Geometry: final body of the model. Coordinates: model frame, mm. Face numbers are marked on the shaded views. Coordinates: 2 decimals unless noted, no trailing zeros. Order: outer loops, then holes, each group sorted by start corner. A loop starts at its lowest first (then second) coordinate and runs counter-clockwise, first axis right, second up. Notation, with made-up numbers: M 62,-12.75 L 90,-12.75 A29 cw 90,9.25 Z; hole C -24,38 d6. An arc over 180 degrees is marked long. Use CSV: the item, a comma, the result in double quotes. Start each with the question number.
1. Section query A-A on x = 266. Return the cut outline in (y, z), and give its area (3 significant figures).
2. First-contact query: P1, Ø10, axis at y = -292.5, z = -432, coming from the +X side; P2, Ø1.5, axis at x = 195, y = -426.5, coming from the -Z side; P3, Ø3, axis at y = 471, z = -355, coming from the -X side. Flat tips, straight axial feed; report the tip coordinate or a pass-through.
3. Material intervals for line 1 (X direction, y = -71, z = -378.5); line 2 (Y direction, x = 176.5, z = -317); line 3 (X direction, y = -426.5, z = -334), sorted ascending.
4. Pull-direction query (Y, two-part tool) for the marked faces 1, 2 and 3; classes: pulls with the +Y half, pulls with the -Y half, needs draft (parallel to the pull), parting line crosses it, or undercut.
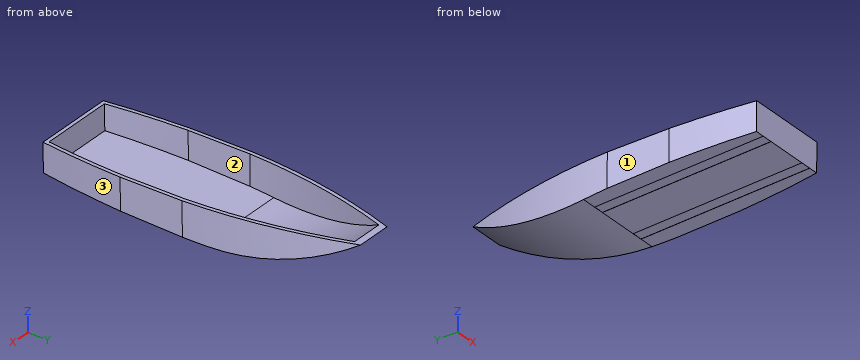
from build123d import *

# Parameters (mm, degrees)
F1_DEPTH = 457.2
F3_DEPTH = 254
F4_T     = 17.78
F5_W     = 50.8
F5_H     = 826.8460257717
F6_DEPTH = 0.508


# Not quite as in the source:
# - a shell that OpenCascade refuses in one call is made with other operations: the cavity is built on its own and cut out


with BuildPart() as f1:
    # F0 (on Right) → F1 (new body)
    with BuildSketch(Plane.YZ):
        with BuildLine():
            Line((288.924485445, -270.4285681248), (-641.1148309708, -283.2744121552))
            Line((-641.1148309708, -283.2744121552), (-641.1148309708, -423.2941567898))
            Line((-641.1148309708, -423.2941567898), (187.4422878027, -442.5629377365))
            ThreePointArc((187.4422878027, -442.5629377365), (523.0417315747, -400.6371692989), (831.9446638759, -262.9282910995))
            Line((831.9446638759, -262.9282910995), (288.924485445, -270.4285681248))
        make_face()
    extrude(amount=F1_DEPTH)

    # F2 (on face) → F3 (cut)
    with BuildSketch(Plane(origin=(0, 3.7895971393, -274.3668944279), x_dir=(1, 0, 0), z_dir=(0, -0.0138108343, 0.9999046259))):
        with BuildLine():
            Line((423.3823697388, -644.965941169), (615.9012913704, -644.965941169))
            Line((615.9012913704, -644.965941169), (483.5176634908, 828.234058831))
            Line((483.5176634908, 828.234058831), (457.2, 61.5478307009))
            ThreePointArc((457.2, 61.5478307009), (455.0788529219, -292.4168742611), (423.3823697388, -644.965941169))
        make_face()
        with BuildLine():
            ThreePointArc((0, 61.5478307009), (43.5944295305, 450.079610673), (142.875, 828.234058831))
            Line((142.875, 828.234058831), (0, 828.234058831))
            Line((0, 828.234058831), (-26.3176634908, 828.234058831))
            Line((-26.3176634908, 828.234058831), (0, 61.5478307009))
        make_face()
        with BuildLine():
            ThreePointArc((33.8176302612, -644.965941169), (2.1211470781, -292.4168742611), (0, 61.5478307009))
            Line((0, 61.5478307009), (-26.3176634908, 828.234058831))
            Line((-26.3176634908, 828.234058831), (-361.6100847721, -644.965941169))
            Line((-361.6100847721, -644.965941169), (33.8176302612, -644.965941169))
        make_face()
        with BuildLine():
            Line((457.2, 61.5478307009), (483.5176634908, 828.234058831))
            Line((483.5176634908, 828.234058831), (457.2, 828.234058831))
            Line((457.2, 828.234058831), (314.325, 828.234058831))
            ThreePointArc((314.325, 828.234058831), (413.6055704695, 450.079610673), (457.2, 61.5478307009))
        make_face()
        Polygon((0, -644.965941169), (-361.6100847721, -644.965941169), (237.2898459435, -852.3167967796), (615.9012913704, -644.965941169), (457.2, -644.965941169), (423.3823697388, -644.965941169), (33.8176302612, -644.965941169), align=None)
    extrude(amount=-F3_DEPTH, mode=Mode.SUBTRACT)

    # F4: shell of thickness 17.78, made by hand


with BuildPart() as f4_core1:
    # F4_t2: copy of F1
    add(f1.part)

    # the walls: a layer under each face that stays
    f4_faces = [f4_core1.faces().sort_by_distance(p)[0] for p in [
        (228.6, 523.0417315747, -400.6371692989),
        (43.5944295305, 455.0197886911, -354.5608330612),
        (413.6055704695, 455.0197886911, -354.5608330612),
        (228.6, -225.8689739056, -432.9510425705),
        (0, -85.1524982143, -356.6467120233),
        (12.0864906617, -438.857755801, -358.0029304556),
        (228.6, -640.1475332924, -353.3067797799),
        (445.1135093383, -438.857755801, -358.0029304556),
        (457.2, -85.1524982143, -356.6467120233),
    ]]
    thicken(f4_faces, amount=-F4_T, mode=Mode.SUBTRACT)


with BuildPart() as f1_1:
    add(f1.part)

    # what is left inside the walls is the cavity
    f4_cavity = [f4_core1.part.solids().sort_by_distance(p)[0] for p in [
        (298.873333, 87.021104, -273.395105),
    ]]
    add(f4_cavity, mode=Mode.SUBTRACT)

    # F5 (on face) → F6 (cut)
    with BuildSketch(Plane(origin=(0, -10.1852834725, -437.9669451445), x_dir=(1, 0, 0), z_dir=(0, -0.0232495407, -0.9997296929))):
        with Locations((103.6994478941, 215.7420070303)):
            Rectangle(F5_W, F5_H)
        with Locations((353.5005521059, 215.7420070303)):
            Rectangle(F5_W, F5_H)
    extrude(amount=-F6_DEPTH, mode=Mode.SUBTRACT)


solid = f1_1.part
Results list:
1,outline,"M -641.11,-283.27 L -639.18,-423.34 L 187.44,-442.56 A1150.36 ccw 831.94,-262.93 L 797.37,-263.41 A1132.58 cw 187.86,-424.79 L -621.64,-405.96 L -623.34,-283.03 Z"
1,area,"28,600 mm²"
2,P1,"stops at x = 455.03"
2,P2,"stops at z = -428.3"
2,P3,"stops at x = 46.33"
3,line 1,"x = 0 to 17.78, 439.42 to 457.2"
3,line 2,"y = -640.65 to -622.87, 697.06 to 737.4"
3,line 3,"x = 11.04 to 28.88, 428.32 to 446.16"
4,face 1,"needs draft"
4,face 2,"undercut"
4,face 3,"pulls with the -Y half"
